Autodesk Inventor part; units mm, degrees
ref_plane "YZ Plane" through (0, 0, 0) normal (1, 0, 0) x (0, 1, 0)
ref_plane "XZ Plane" through (0, 0, 0) normal (0, 1, 0) x (-1, 0, 0)
ref_plane "XY Plane" through (0, 0, 0) normal (0, 0, 1) x (1, 0, 0)
sketch "Skizze2" plane through (0, 0, 0) normal (0, 1, 0) x (-1, 0, 0)
  line L0 (0, 514) -> (0, -212) construction
  line L1 (-35, 0) -> (35, 0)
  line L2 (35, 0) -> (35, 1020)
  line L3 (35, 1020) -> (-35, 1020)
  line L4 (-35, 1020) -> (-35, 0)
  point P0 (0, 0)
  dimension "breite" = 70
  dimension "laenge" = 1020
extrude "Extrusion1" add sketch "Skizze2" along normal blind 4
sketch "Skizze3" plane through (0, 0, 0) normal (0, -1, 0) x (1, 0, 0)
  line L0 (35, 0) -> (-35, 0)
  line L1 (35, 1020) -> (35, 0)
  line L2 (-35, 1020) -> (35, 1020)
  line L3 (-35, 0) -> (-35, 1020)
  line L4 (-35, 1020) -> (35, 1020)
  line L5 (35, 0) -> (-35, 0)
  line L6 (-25, 1020) -> (25, 1020)
  line L7 (25, 1020) -> (25, 0)
  line L8 (25, 0) -> (-25, 0)
  line L9 (-25, 0) -> (-25, 1020)
  line L10 (0, 1159.0325) -> (0, -216) construction
  point P0 (0, 0)
  dimension "d4" = 50
extrude "Extrusion2" add sketch "Skizze3" along normal blind 14 contours L0 L9 L2 L7
sketch "Skizze4" plane through (0, -14, 0) normal (0, -1, 0) x (1, 0, 0)
  line L0 (-25, 1020) -> (-25, 0)
  line L1 (-25, 0) -> (25, 0)
  line L2 (25, 0) -> (25, 1020)
  line L3 (25, 1020) -> (-25, 1020)
  line L4 (-8.5, 995) -> (8.5, 995)
  line L5 (8.5, 995) -> (8.5, 25)
  line L6 (8.5, 25) -> (-8.5, 25)
  line L7 (-8.5, 25) -> (-8.5, 995)
  line L8 (0, -47) -> (0, 1281) construction
  line L9 (-397, 510) -> (541, 510) construction
  line L10 (35, 1020) -> (35, 0)
  line L11 (-25, 0) -> (25, 0)
  line L12 (25, 0) -> (25, 25)
  line L13 (25, 25) -> (-25, 25)
  line L14 (-25, 25) -> (-25, 0)
  line L15 (-25, 1020) -> (25, 1020)
  line L16 (25, 1020) -> (25, 995)
  line L17 (25, 995) -> (-25, 995)
  line L18 (-25, 995) -> (-25, 1020)
  line L19 (-24, 1) -> (26, 1)
  line L20 (26, 1021) -> (-24, 1021)
  line L21 (-7.5, 996) -> (9.5, 996)
  line L22 (9.5, 26) -> (-7.5, 26)
  line L23 (-24, 1) -> (26, 1)
  line L24 (26, 1) -> (26, 26)
  line L25 (26, 26) -> (-24, 26)
  line L26 (-24, 26) -> (-24, 1)
  line L27 (-24, 1021) -> (26, 1021)
  line L28 (26, 1021) -> (26, 996)
  line L29 (26, 996) -> (-24, 996)
  line L30 (-24, 996) -> (-24, 1021)
  point P0 (0, 0)
  point P1 (1, 1)
  point P2 (36, 1021)
  point P3 (36, 1)
  dimension "d8" = 25
  dimension "d9" = 510
  dimension "d10" = 35
  dimension "d11" = 17
  dimension "d14" = 25
  dimension "d15" = 17
extrude "Extrusion3" cut sketch "Skizze4" against normal blind 10 contours L4 L5 L22 L25 L7 | L25 L22 L5 L6 L7
sketch "Skizze6" plane through (0, -14, 0) normal (0, -1, 0) x (1, 0, 0)
  line L0 (-25, 0) -> (25, 0)
  line L1 (25, 1020) -> (-25, 1020)
  line L2 (-8.5, 995) -> (8.5, 995)
  line L3 (8.5, 25) -> (-8.5, 25)
  line L4 (-25, 0) -> (25, 0)
  line L5 (25, 0) -> (25, 25)
  line L6 (25, 25) -> (-25, 25)
  line L7 (-25, 25) -> (-25, 0)
  line L8 (-25, 1020) -> (25, 1020)
  line L9 (25, 1020) -> (25, 995)
  line L10 (25, 995) -> (-25, 995)
  line L11 (-25, 995) -> (-25, 1020)
  point P0 (0, 0)
  point P1 (0, 0)
  point P2 (35, 1020)
  point P3 (35, 0)
  dimension "d16" = 25
  dimension "d17" = 17
extrude "Extrusion4" cut sketch "Skizze6" against normal blind 3
sketch "Skizze7" plane through (0, 0, 0) normal (0, -1, 0) x (1, 0, 0)
  line L0 (-25, 0) -> (-25, 1020)
  line L1 (-35, 1020) -> (-25, 1020)
  line L2 (-35, 0) -> (-35, 1020)
  line L3 (-25, 0) -> (-35, 0)
  line L4 (25, 1020) -> (25, 0)
  line L5 (35, 0) -> (25, 0)
  line L6 (35, 1020) -> (35, 0)
  line L7 (25, 1020) -> (35, 1020)
  line L8 (0, 1058) -> (0, -187) construction
  line L9 (-30, 1012) -> (-30, 5) construction
  point P0 (0, 0)
  point P1 (-30, 760.25)
  point P2 (-30, 508.5)
  point P3 (-30, 256.75)
  point P4 (30, 1012)
  point P5 (30, 5)
  point P6 (30, 760.25)
  point P7 (30, 508.5)
  point P8 (30, 256.75)
  dimension "d20" = 5
  dimension "d21" = 8
  dimension "d22" = 5
  dimension "d23" = 5
  dimension "d26" = 251.75
  dimension "d27" = 503.5
  dimension "d28" = 755.25
hole "Bohrung1" at (-30, 0, 1012) at (-30, 0, 5) at (-30, 0, 760.25) at (-30, 0, 508.5) at (-30, 0, 256.75) at (30, 0, 1012) at (30, 0, 760.25) at (30, 0, 508.5) at (30, 0, 256.75) at (30, 0, 5) direction (0, 1, 0) diameter 8 depth 1
equation "\"d9\" = 0.5 * laenge"
equation "\"d10\" = 0.5 * breite"
properties part number "Wiper-Woodconstruction" material "Holz (Birke)"
CAD build for the part. Positions are in the model's coordinates, mm. A direction names the side the tool comes from. Coordinates: 2 decimals unless noted, no trailing zeros. Order: outer loops, then holes, each group sorted by start corner. A loop starts at its lowest first (then second) coordinate and runs counter-clockwise, first axis right, second up.
(1) Mould opens along X. For faces 3 (the face through (0, -4, 517)), 4 (the face through (0, -11, 1008)) say: released by +X, released by -X, zero draft, split by the parting line, or undercut.
Solution:
face 3: undercut
face 4: zero draft
(2) Pin check, flat tips, straight feed: pin 1 Ø7 at (y, z) = (-10, 576) entering from +X; pin 2 Ø2.5 at (x, z) = (-28.5, 762) entering from -Y; pin 3 Ø1.5 at (y, z) = (-9, 103.5) entering from -X; pin 4 Ø8 at (x, y) = (-8.5, -9.5) entering from -Z. Stop position of each tip, or through.
Solution:
pin 1: stops at x = 25
pin 2: stops at y = 1
pin 3: stops at x = -25
pin 4: stops at z = 0
(3) Which spindle directions (+Z, -Z, +X, -X, +Y, -Y) get a long thin tool onto all of the face, cutting with end or side? Do faces 1 (the face through (-17, -14, 517)), 2 (the face through (0, -11, 13)). Say none if no direction does.
Solution:
face 1: +Z, -Z, +X, -X, -Y
face 2: -Z, +X, -X, -Y
(4) Drill centre lines: L1, parallel to X at y = 0.4, z = 760.25; L2, parallel to Z at x = 30, y = 0.85; L3, parallel to X at y = -9.5, z = 395. Where is each one in solid material? Low to high.
Solution:
L1: x = -35 to -34, -26 to 26, 34 to 35
L2: z = 0 to 1, 9 to 252.75, 260.75 to 504.5, 512.5 to 756.25, 764.25 to 1008, 1016 to 1020
L3: x = -25 to -8.5, 8.5 to 25
(5) Saw through at B-B, the plane z = 733. Write the cut outline in (x, y).
Solution:
outline: (-35, 0) - (-25, 0) - (-25, -14) - (-8.5, -14) - (-8.5, -4) - (8.5, -4) - (8.5, -14) - (25, -14) - (25, 0) - (35, 0) - (35, 4) - (-35, 4) - close
(6) Saw through at A-A, the plane y = -8.25. Write the cut outline in (x, z).
Solution:
outline: (-25, 0) - (25, 0) - (25, 1020) - (-25, 1020) - close; hole (-8.5, 25) - (8.5, 25) - (8.5, 995) - (-8.5, 995) - close
